Autodesk Inventor part; units mm, degrees
ref_plane "YZ Plane" through (0, 0, 0) normal (1, 0, 0) x (0, 1, 0)
ref_plane "XZ Plane" through (0, 0, 0) normal (0, 1, 0) x (-1, 0, 0)
ref_plane "XY Plane" through (0, 0, 0) normal (0, 0, 1) x (1, 0, 0)
sketch "Sketch1" plane through (0, 0, 0) normal (0, 1, 0) x (-1, 0, 0)
  line L0 (-106, 106) -> (106, 106)
  line L1 (106, 106) -> (106, -106)
  line L2 (106, -106) -> (-106, -106)
  line L3 (-106, -106) -> (-106, 106)
  line L4 (-106, 106) -> (106, -106) construction
  line L5 (106, 106) -> (-106, -106) construction
  point P0 (0, 0)
  dimension "d0" = 212
  dimension "d1" = 212
extrude "Extrusion1" add sketch "Sketch1" along normal blind 3
sketch "Sketch2" plane through (0, 3, 0) normal (0, 1, 0) x (1, 0, 0)
  line L0 (-106, 106) -> (-106, -106)
  line L1 (106, 106) -> (-106, 106)
  line L2 (-106, -106) -> (-103, -106)
  line L3 (-103, -106) -> (-103, 106)
  line L4 (-103, 106) -> (-106, 106)
  line L5 (-106, 106) -> (-106, -106)
  line L6 (106, -106) -> (106, 106)
  line L7 (-106, -106) -> (106, -106)
  line L8 (106, 106) -> (103, 106)
  line L9 (103, 106) -> (103, -106)
  line L10 (103, -106) -> (106, -106)
  line L11 (106, -106) -> (106, 106)
  line L12 (106, 106) -> (-106, 106)
  line L13 (-106, 106) -> (-106, 103)
  line L14 (-106, 103) -> (106, 103)
  line L15 (106, 103) -> (106, 106)
  line L16 (-106, -106) -> (106, -106)
  line L17 (106, -106) -> (106, -103)
  line L18 (106, -103) -> (-106, -103)
  line L19 (-106, -103) -> (-106, -106)
  point P0 (0, 0)
  point P1 (-103, 103)
  point P2 (103, 103)
  point P3 (103, -103)
  point P4 (-103, -103)
  dimension "d4" = 3
  dimension "d5" = 3
  dimension "d6" = 3
  dimension "d7" = 3
extrude "Extrusion2" add sketch "Sketch2" along normal blind 300 contours L1 L3 L14 L0 | L14 L3 L18 L0 | L1 L9 L14 L3 | L18 L3 L2 L0 | L1 L6 L14 L9 | L18 L9 L7 L3 | L14 L6 L18 L9 | L18 L6 L7 L9
sketch "Sketch3" plane through (-103, 3, 103) normal (1, 0, 0) x (0, 0, -1)
  line L0 (0, 0) -> (0, 300)
  line L1 (206, 0) -> (206, 300)
  line L2 (0, 300) -> (206, 300)
  line L3 (206, 300) -> (206, 297)
  line L4 (206, 297) -> (0, 297)
  line L5 (0, 297) -> (0, 300)
  point P0 (103, -3)
  dimension "d10" = 3
extrude "Extrusion3" add sketch "Sketch3" along normal up to surface (209 mm away)
sketch "Sketch4" plane through (-106, 0, -106) normal (-1, 0, 0) x (0, 0, 1)
  line L0 (3, 3) -> (209, 3)
  line L1 (3, 3) -> (209, 3)
  line L2 (209, 3) -> (209, 93)
  line L3 (209, 93) -> (3, 93)
  line L4 (3, 93) -> (3, 3)
  point P0 (106, 0)
  dimension "d13" = 90
extrude "Extrusion4" cut sketch "Sketch4" against normal blind 10
sketch "Sketch5" plane through (-106, 0, 106) normal (0, 0, 1) x (1, 0, 0)
  line L0 (0, 93) -> (3, 93)
  line L1 (0, 3) -> (209, 3)
  line L2 (0, 93) -> (209, 93)
  line L3 (209, 93) -> (209, 3)
  line L4 (209, 3) -> (0, 3)
  line L5 (0, 3) -> (0, 93)
  point P0 (106, 0)
extrude "Extrusion5" cut sketch "Sketch5" against normal blind 10
sketch "Sketch6" plane through (106, 0, 106) normal (1, 0, 0) x (0, 0, -1)
  line L0 (3, 93) -> (209, 93)
  line L1 (0, 303) -> (212, 303)
  line L2 (0, 0) -> (0, 303)
  line L3 (0, 0) -> (212, 0)
  line L4 (212, 0) -> (212, 303)
  line L5 (212, 0) -> (0, 0)
  line L6 (0, 0) -> (0, 93)
  line L7 (0, 93) -> (212, 93)
  line L8 (212, 93) -> (212, 0)
  line L9 (212, 93) -> (0, 0) construction
  line L10 (0, 93) -> (0, 3) construction
  line L11 (0, 93) -> (212, 0) construction
  line L12 (131, 71.5) -> (81, 71.5)
  line L13 (81, 71.5) -> (81, 21.5)
  line L14 (81, 21.5) -> (131, 21.5)
  line L15 (131, 21.5) -> (131, 71.5)
  line L16 (131, 71.5) -> (81, 21.5) construction
  line L17 (81, 71.5) -> (131, 21.5) construction
  point P0 (106, 0)
  point P1 (106, 46.5)
  dimension "d18" = 50
  dimension "d19" = 50
extrude "Extrusion6" cut sketch "Sketch6" against normal blind 10 contours L15 L14 L13 L12
properties part number "Hot Box Case" material "Polycarbonate, Smoke"
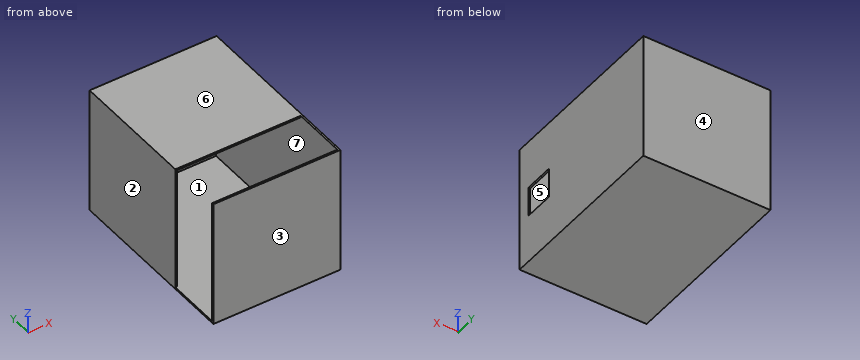
Could you check a few things on this model? Use its own coordinates, in mm. Face numbers are marked on the shaded views. A direction names the side the tool comes from. Coordinates: 2 decimals unless noted, no trailing zeros. Write each loop counter-clockwise with the first axis right and the second up, starting at its lowest first coordinate (ties: lowest second). Pieces come first, ordered by that corner, then holes. Notation, with made-up numbers: (43, 7) -> (83, 7) arc R31 ccw to (83, 35) -> close; hole circle Ø4 at (-31.5, 89). An arc over 180 degrees is marked (long way). Return JSON: item names as keys, results as strings.
(1) I need wall thicknesses on L1, parallel to Y at x = 77.5, z = 74; L2, parallel to Z at x = 88.5, y = 139. Which ranges of each line are inside material? Lowest first, please.
Numbers:
{"L1": "y = 0 to 3, 300 to 303", "L2": "z = -106 to -103, 103 to 106"}
(2) I'm going to push a flat-ended pin straight in: pin 1 (2.5 mm diameter, centred on x = 104.5, z = -12, fed in from -Y). Where does the tip first touch, or does it pass through?
Numbers:
{"pin 1": "stops at y = 0"}
(3) Imagine slicing it at D-D, the plane y = 225. Please give me the cut outline in (x, z), then the cut area to 3 significant figures.
Numbers:
{"outline": "(-106, -106) -> (106, -106) -> (106, 106) -> (-106, 106) -> close; hole (-103, -103) -> (103, -103) -> (103, 103) -> (-103, 103) -> close", "area": "2,510 mm2"}
(4) Which directions (+Z, -Z, +X, -X, +Y, -Y) give clear straight access to the entire face, cutting with the end or side of a thin tool? Please do the marked faces 5, 6 and 7.
Numbers:
{"face 5": "+Z, -X", "face 6": "+Z, +X, -X, +Y, -Y", "face 7": "none"}
(5) We'd pull the mould along Y, two halves only. Please class the marked faces 1, 2, 3 and 4: +Y half, -Y half, draft (parallel to the pull), parting line (faces both ways), or undercut.
Numbers:
{"face 1": "undercut", "face 2": "draft", "face 3": "-Y half", "face 4": "+Y half"}
(6) Imagine slicing it at A-A, the plane y = 45.5. Please give me the cut outline in (x, z).
Numbers:
{"outline": "(-106, -106) -> (106, -106) -> (106, -25) -> (103, -25) -> (103, -103) -> (-106, -103) -> close; (103, 25) -> (106, 25) -> (106, 106) -> (103, 106) -> close"}
(7) Imagine slicing it at C-C, the plane x = -82.5. Please give me the cut outline in (y, z), then the cut area to 3 significant figures.
Numbers:
{"outline": "(0, -106) -> (303, -106) -> (303, 106) -> (93, 106) -> (93, 103) -> (300, 103) -> (300, -103) -> (3, -103) -> (3, 106) -> (0, 106) -> close", "area": "2,780 mm2"}
(8) Imagine slicing it at B-B, the plane z = -0.5. Please give me the cut outline in (x, y), then the cut area to 3 significant figures.
Numbers:
{"outline": "(-106, 0) -> (106, 0) -> (106, 21.5) -> (103, 21.5) -> (103, 3) -> (-106, 3) -> close; (-106, 93) -> (-103, 93) -> (-103, 300) -> (103, 300) -> (103, 71.5) -> (106, 71.5) -> (106, 303) -> (-106, 303) -> close", "area": "2,630 mm2"}
